from build123d import *

# Parameters (mm, degrees)
SKETCH_1_W          = 12.3
SKETCH_1_H          = 11.3
EXTRUDE_1_DEPTH     = 2.5
SKETCH_2_W          = 1.5
SKETCH_2_H          = 11.3
EXTRUDE_2_DEPTH     = 4.35
SKETCH_5_W          = 9.3
SKETCH_5_H          = 11.5
CUT_EXTRUDE_1_DEPTH = 1
SKETCH_8_W          = 1.6
SKETCH_8_H          = 11.3
EXTRUDE_5_DEPTH     = 0.8
SKETCH_9_W          = 1.6
SKETCH_9_H          = 11.3
EXTRUDE_6_DEPTH     = 0.8
FILLET_7_R          = 0.8
FILLET_8_R          = 0.3


with BuildPart() as part:
    # 스케치1 → 보스-돌출1 (new body)
    with BuildSketch(Plane.XY):
        Rectangle(SKETCH_1_W, SKETCH_1_H)
    extrude(amount=EXTRUDE_1_DEPTH)

    # 스케치2 → 보스-돌출2 (add)
    with BuildSketch(Plane.XY.offset(2.5)):
        with Locations((-5.4, 0)):
            Rectangle(SKETCH_2_W, SKETCH_2_H)
        with Locations((5.4, 0)):
            Rectangle(SKETCH_2_W, SKETCH_2_H)
    extrude(amount=EXTRUDE_2_DEPTH)

    # 스케치5 → 컷-돌출1 (cut)
    with BuildSketch(Plane.XY.offset(2.5)):
        Rectangle(SKETCH_5_W, SKETCH_5_H)
    extrude(amount=-CUT_EXTRUDE_1_DEPTH, mode=Mode.SUBTRACT)

    # 스케치8 → 보스-돌출5 (add)
    with BuildSketch(Plane(origin=(-4.65, 0, 0), x_dir=(0, 0, -1), z_dir=(1, 0, 0))):
        with Locations((-6.05, 0)):
            Rectangle(SKETCH_8_W, SKETCH_8_H)
    extrude(amount=EXTRUDE_5_DEPTH)

    # 스케치9 → 보스-돌출6 (add)
    with BuildSketch(Plane.ZY.offset(-4.65)):
        with Locations((6.05, 0)):
            Rectangle(SKETCH_9_W, SKETCH_9_H)
    extrude(amount=EXTRUDE_6_DEPTH)

    # 필렛7
    fillet_7_edges = [part.edges().sort_by_distance(p)[0] for p in [
        (3.85, 0, 6.85),
        (-3.85, 0, 6.85),
        (3.85, 0, 5.25),
        (-3.85, 0, 5.25),
    ]]
    fillet(fillet_7_edges, radius=FILLET_7_R - 0.0001)  # a hair under: the kernel refuses the full size

    # 필렛8
    fillet_8_edges = [part.edges().sort_by_distance(p)[0] for p in [
        (4.65, 0, 1.5),
        (-4.65, 0, 1.5),
    ]]
    fillet(fillet_8_edges, radius=FILLET_8_R)


solid = part.part
Read the model definition and answer for the solid it produces. Units are mm, in the model's axes. A direction names the side the tool comes from. Round coordinates to 2 decimals unless told otherwise and drop trailing zeros. Order: outer loops, then holes, each group sorted by start corner. A loop starts at its lowest first (then second) coordinate and runs counter-clockwise, first axis right, second up. Notation, with made-up numbers: (-9, 14.25) - (6, 14.25) arc R19 ccw to (6, 33.25) - close; hole circle Ø7 at (14.5, 0). An arc over 180 degrees is marked (long way). Use one line per item in the form item = value. Start each with the question number.
(1) Determine the mould class of faces 1 (the face through (-5, 0, 6.85)), 2 (the face through (-6.15, 0, 3)), 3 (the face through (-4.65, 0, 4)) for opening direction Z: +Z half, -Z half, draft (parallel to the pull), parting line (faces both ways), or undercut.
(2) The part is cut by section A-A (z = 2). Give the vertices of the cut face in (x, y).
(3) The part is cut by section C-C (x = 4). Give the vertices of the cut face in (y, z), then the cut area to 3 significant figures.
(4) For faces 4 (the face through (0, -5.65, 1)), 5 (the face through (4.65, 0, 4)), determine the directions among +Z, -Z, +X, -X, +Y, -Y from which every point of the face is accessible in a straight line to the end or side of a thin tool.
(5) The part is cut by section D-D (x = -1.25). Give the vertices of the cut face in (y, z).
(6) Find the intervals of material crossed by line 1 along X through (y, z) = (-1.75, 3.75); line 2 along X through (y, z) = (-2.75, 6.75); line 3 along Z through (x, y) = (0.75, 1.5), in increasing order. Write a range as from..to.
Checked values:
q1.face_1 = +Z half
q1.face_2 = draft
q1.face_3 = undercut
q2.outline = (-6.15, -5.65) - (-4.65, -5.65) - (-4.65, 5.65) - (-6.15, 5.65) - close; (4.65, -5.65) - (6.15, -5.65) - (6.15, 5.65) - (4.65, 5.65) - close
q3.outline = (-5.65, 0) - (5.65, 0) - (5.65, 1.5) - (-5.65, 1.5) - close; (-5.65, 5.58) - (5.65, 5.58) - (5.65, 6.52) - (-5.65, 6.52) - close
q3.area = 27.5 mm^2
q4.face_4 = +Z, -Z, +X, -X, -Y
q4.face_5 = +Y, -Y
q5.outline = (-5.65, 0) - (5.65, 0) - (5.65, 1.5) - (-5.65, 1.5) - close
q6.line_1 = -6.15..-4.65, 4.65..6.15
q6.line_2 = -6.15..-4.26, 4.26..6.15
q6.line_3 = 0..1.5
